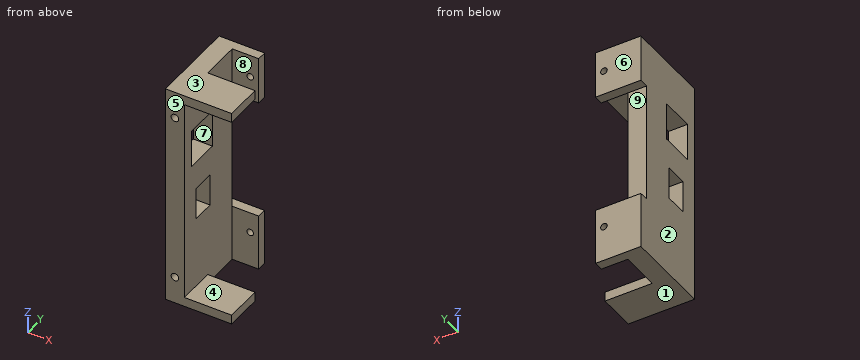
```python
from build123d import *

# Parameters (mm, degrees)
SKETCH1_W      = 10
SKETCH1_H      = 119
EXTRUDE1_DEPTH = 46
SKETCH2_W      = 5
SKETCH2_H      = 20
EXTRUDE2_DEPTH = 35
SKETCH3_W      = 64
SKETCH3_H      = 5
SKETCH3_W_2    = 17
SKETCH3_H_2    = 12
SKETCH3_W_3    = 20
SKETCH3_H_3    = 18
EXTRUDE3_DEPTH = 30
SKETCH4_W      = 25
SKETCH4_H      = 5
SKETCH4_W_2    = 30
EXTRUDE4_DEPTH = 14
SKETCH5_R      = 1.75
EXTRUDE5_DEPTH = 5
SKETCH7_R      = 2
EXTRUDE6_DEPTH = 10


with BuildPart() as part:
    # Sketch1 → Extrude1 (new body)
    with BuildSketch(Plane(origin=(0, 0, 0), x_dir=(1, 0, 0), z_dir=(0, 1, 0))):
        Rectangle(SKETCH1_W, SKETCH1_H)
    extrude(amount=EXTRUDE1_DEPTH)

    # Sketch2 → Extrude2 (add)
    with BuildSketch(Plane.ZY.offset(5)):
        with Locations((-57, 10)):
            Rectangle(SKETCH2_W, SKETCH2_H)
        with Locations((57, 10)):
            Rectangle(SKETCH2_W, SKETCH2_H)
    extrude(amount=-EXTRUDE2_DEPTH)

    # Sketch3 → Extrude3 (cut)
    with BuildSketch(Plane.ZY.offset(5)):
        with Locations((2.5, 43.5)):
            Rectangle(SKETCH3_W, SKETCH3_H)
        with Locations((-8, 16)):
            Rectangle(SKETCH3_W_2, SKETCH3_H_2)
        with Locations((25.5, 15)):
            Rectangle(SKETCH3_W_3, SKETCH3_H_3)
    extrude(amount=-EXTRUDE3_DEPTH, mode=Mode.SUBTRACT)

    # Sketch4 → Extrude4 (add)
    with BuildSketch(Plane(origin=(5, 0, 0), x_dir=(0, 0, -1), z_dir=(1, 0, 0))):
        with Locations((-47, 43.5)):
            Rectangle(SKETCH4_W, SKETCH4_H)
        with Locations((44.5, 43.5)):
            Rectangle(SKETCH4_W_2, SKETCH4_H)
    extrude(amount=EXTRUDE4_DEPTH)

    # Sketch5 → Extrude5 (cut)
    with BuildSketch(Plane(origin=(0, 46, 0), x_dir=(1, 0, 0), z_dir=(0, 1, 0))):
        with Locations(Location((14.5, -47.5, 0), (0, 0, 270))):
            Circle(SKETCH5_R)
        with Locations(Location((14.5, 40.5, 0), (0, 0, 270))):
            Circle(SKETCH5_R)
    extrude(amount=-EXTRUDE5_DEPTH, mode=Mode.SUBTRACT)

    # Sketch7 → Extrude6 (cut)
    with BuildSketch(Plane.XZ):
        with Locations(Location((0, 45, 0), (0, 0, 270))):
            Circle(SKETCH7_R)
        with Locations(Location((0, -45, 0), (0, 0, 270))):
            Circle(SKETCH7_R)
    extrude(amount=-EXTRUDE6_DEPTH, mode=Mode.SUBTRACT)


solid = part.part
```
Verification items for the finished model (mm, model axes). Face numbers are marked on the shaded views. A direction names the side the tool comes from. Give positions to 0.01 mm unless a question says otherwise; leave off trailing zeros. Order: outer loops, then holes, each group sorted by start corner. A loop starts at its lowest first (then second) coordinate and runs counter-clockwise, first axis right, second up. Notation, with made-up numbers: (-35, 41.25) - (-15, 41.25) arc R17 ccw to (-15, 68.25) - close; hole circle Ø10 at (53, 36). An arc over 180 degrees is marked (long way). Answer as CSV lines item,"result". Start each with the question number.
Item 1: Section check B-B, the plane x = 8.5. Record the boundary of the cut face in (y, z).
Item 2: Section check A-A, the plane z = 30.5. Record the boundary of the cut face in (x, y).
Item 3: Gauge pin test, flat ends, axial feed: pin 1 (11 mm diameter, centred on x = 0, z = -9, fed in from +Y); pin 2 (2.5 mm diameter, centred on y = 43, z = -47, fed in from +X); pin 3 (4 mm diameter, centred on x = 22.5, z = 58, fed in from +Y). Record the tip position at first contact, or that the pin passes through.
Item 4: Material ranges on L1, parallel to Z at x = 3, y = 17.5; L2, parallel to Y at x = 0, z = 19; L3, parallel to X at y = 44.55, z = -40.5, recorded low to high.
Item 5: Access from +Z, -Z, +X, -X, +Y, -Y to the whole of each face (thin tool, end or side, straight path). Record for the marked faces 5, 6, 7, 8 and 9.
Item 6: Mould release check, pull along Z, two halves, no side actions. Record for the marked faces 1, 2, 3 and 4: released by +Z, released by -Z, zero draft, split by the parting line, or undercut.
Item 7: Section check D-D, the plane x = 14.5. Record the boundary of the cut face in (y, z).
Item 8: Section check C-C, the plane y = 17.5. Record the boundary of the cut face in (x, z).
Filled in:
1,outline,"(0, -59.5) - (20, -59.5) - (20, -54.5) - (0, -54.5) - close; (0, 54.5) - (20, 54.5) - (20, 59.5) - (0, 59.5) - close; (41, -59.5) - (46, -59.5) - (46, -29.5) - (41, -29.5) - close; (41, 34.5) - (46, 34.5) - (46, 59.5) - (41, 59.5) - close"
2,outline,"(-5, 0) - (5, 0) - (5, 6) - (-5, 6) - close; (-5, 24) - (5, 24) - (5, 41) - (-5, 41) - close"
3,pin 1,"y = 41"
3,pin 2,"x = 19"
3,pin 3,"y = 20"
4,L1,"-59.5 to -16.5, 0.5 to 15.5, 35.5 to 59.5"
4,L2,"0 to 6, 24 to 41"
4,L3,"-5 to 12.75, 16.25 to 19"
5,face 5,"+Z, -Z, +X, -X, -Y"
5,face 6,"+Z, -Z, +X, -X, +Y"
5,face 7,"+X, -X"
5,face 8,"+Z, -Z, +X"
5,face 9,"+X, -X, +Y"
6,face 1,"released by -Z"
6,face 2,"zero draft"
6,face 3,"released by +Z"
6,face 4,"undercut"
7,outline,"(0, -59.5) - (20, -59.5) - (20, -54.5) - (0, -54.5) - close; (0, 54.5) - (20, 54.5) - (20, 59.5) - (0, 59.5) - close; (41, -59.5) - (46, -59.5) - (46, -42.25) - (41, -42.25) - close; (41, -38.75) - (46, -38.75) - (46, -29.5) - (41, -29.5) - close; (41, 34.5) - (46, 34.5) - (46, 45.75) - (41, 45.75) - close; (41, 49.25) - (46, 49.25) - (46, 59.5) - (41, 59.5) - close"
8,outline,"(-5, -59.5) - (30, -59.5) - (30, -54.5) - (5, -54.5) - (5, -16.5) - (-5, -16.5) - close; (-5, 0.5) - (5, 0.5) - (5, 15.5) - (-5, 15.5) - close; (-5, 35.5) - (5, 35.5) - (5, 54.5) - (30, 54.5) - (30, 59.5) - (-5, 59.5) - close"
